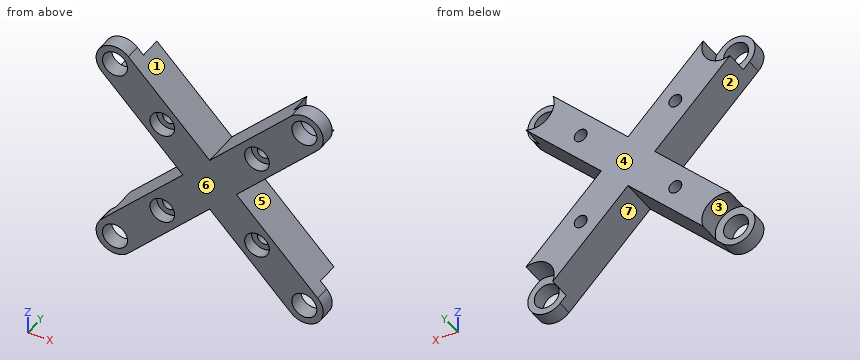
```python
from build123d import *

# Parameters (mm, degrees)
EXTRUDE1_DEPTH                 = 10
CBORE_FOR_M6_SHCS2_D           = 6.6
CBORE_FOR_M6_SHCS2_CBORE_D     = 11
CBORE_FOR_M6_SHCS2_CBORE_DEPTH = 6
LPATTERN1_COUNT                = 2
LPATTERN1_PITCH                = 50
LPATTERN1_COUNT_DIR2           = 2
LPATTERN1_PITCH_DIR2           = 50
CBORE_FOR_M3_SHCS1_D           = 3.4
CBORE_FOR_M3_SHCS1_CBORE_D     = 6.5
CBORE_FOR_M3_SHCS1_CBORE_DEPTH = 3
LPATTERN2_COUNT                = 2
LPATTERN2_PITCH                = 25
LPATTERN2_COUNT_DIR2           = 2
LPATTERN2_PITCH_DIR2           = 25


with BuildPart() as part:
    # Sketch1 → Extrude1 (new body)
    with BuildSketch(Plane(origin=(0, 0, 0), x_dir=(1, 0, 0), z_dir=(0, 1, 0))):
        with BuildLine():
            Line((7.071067812, 0), (28.535533906, 21.464466094))
            ThreePointArc((28.535533906, 21.464466094), (28.535533906, 28.535533906), (21.464466094, 28.535533906))
            Line((21.464466094, 28.535533906), (0, 7.071067812))
            Line((0, 7.071067812), (-21.464466094, 28.535533906))
            ThreePointArc((-21.464466094, 28.535533906), (-28.535533906, 28.535533906), (-28.535533906, 21.464466094))
            Line((-28.535533906, 21.464466094), (-7.071067812, 0))
            Line((-7.071067812, 0), (-28.535533906, -21.464466094))
            ThreePointArc((-28.535533906, -21.464466094), (-28.535533906, -28.535533906), (-21.464466094, -28.535533906))
            Line((-21.464466094, -28.535533906), (0, -7.071067812))
            Line((0, -7.071067812), (21.464466094, -28.535533906))
            ThreePointArc((21.464466094, -28.535533906), (28.535533906, -28.535533906), (28.535533906, -21.464466094))
            Line((28.535533906, -21.464466094), (7.071067812, 0))
        make_face()
    extrude(amount=EXTRUDE1_DEPTH)

    # CBORE for M6 SHCS2 (through all)
    with Locations(Plane(origin=(-25, 10, -25), x_dir=(0, 0, 1), z_dir=(0, 1, 0))):
        with Locations((0, 0)):
            cbore_for_m6_shcs2 = CounterBoreHole(CBORE_FOR_M6_SHCS2_D / 2, CBORE_FOR_M6_SHCS2_CBORE_D / 2, CBORE_FOR_M6_SHCS2_CBORE_DEPTH)

    # LPattern1: CBORE for M6 SHCS2 2 × 2
    with Locations(*[(i * LPATTERN1_PITCH, 0, j * LPATTERN1_PITCH_DIR2) for i in range(LPATTERN1_COUNT) for j in range(LPATTERN1_COUNT_DIR2) if (i, j) != (0, 0)]):
        add(cbore_for_m6_shcs2, mode=Mode.SUBTRACT)

    # CBORE for M3 SHCS1 (through all)
    with Locations(Plane(origin=(-12.5, 0, 12.5), x_dir=(0, 0, -1), z_dir=(0, -1, 0))):
        with Locations((0, 0)):
            cbore_for_m3_shcs1 = CounterBoreHole(CBORE_FOR_M3_SHCS1_D / 2, CBORE_FOR_M3_SHCS1_CBORE_D / 2, CBORE_FOR_M3_SHCS1_CBORE_DEPTH)

    # LPattern2: CBORE for M3 SHCS1 2 × 2
    with Locations(*[(i * LPATTERN2_PITCH, 0, -j * LPATTERN2_PITCH_DIR2) for i in range(LPATTERN2_COUNT) for j in range(LPATTERN2_COUNT_DIR2) if (i, j) != (0, 0)]):
        add(cbore_for_m3_shcs1, mode=Mode.SUBTRACT)


solid = part.part
```
Model file for the job. Use its own axes, mm. Face numbers are marked on the shaded views. A direction names the side the tool comes from. Coordinates: 2 decimals unless noted, no trailing zeros. Order: outer loops, then holes, each group sorted by start corner. A loop starts at its lowest first (then second) coordinate and runs counter-clockwise, first axis right, second up. Notation, with made-up numbers: (63, 44.25) - (114, 44.25) arc R22 cw to (114, 63.25) - close; hole circle Ø8 at (64.5, -40). An arc over 180 degrees is marked (long way). Return JSON: item names as keys, results as strings. Group by question number.
1) Saw through at D-D, the plane z = -17.5. Write the cut outline in (x, y), plus the area to 3 significant figures.
2) Flat gauge pins, fed straight in: P1, Ø3, axis at x = -27, z = -25.5, coming from the +Y side; P2, Ø5.5, axis at x = 12.5, z = 12.5, coming from the -Y side; P3, Ø1.5, axis at x = 14, y = 6, coming from the +Z side. Where does each tip first touch, or does it go through?
3) Mould opens along X. For the marked faces 5, 6 and 7 say: released by +X, released by -X, zero draft, split by the parting line, or undercut.
4) Probe line 1 (X direction, y = 3.05, z = -25); line 2 (X direction, y = 1.1, z = -12.5); line 3 (Z direction, x = -13, y = 0.5). List the from-to ranges inside material, lowest first. Write a range as from..to.
5) Saw through at B-B, the plane x = 12.5. Write the cut outline in (y, z).
6) Saw through at A-A, the plane z = 25. Write the cut outline in (x, y), plus the area to 3 significant figures.
7) Tool access for the marked faces 1, 2, 3 and 4: list every direction of +Z, -Z, +X, -X, +Y, -Y with a clear straight run to the whole face (end or side of a thin tool).
8) Saw through at C-C, the plane y = 5.5. Write the cut outline in (x, z), plus the area to 3 significant figures.
Values found:
{
 "1": {"outline": "(-24.57, 0) - (-10.43, 0) - (-10.43, 10) - (-24.57, 10) - close; (10.43, 0) - (24.57, 0) - (24.57, 10) - (10.43, 10) - close", "area": "283 mm²"},
 "2": {"P1": "stops at y = 4", "P2": "stops at y = 3", "P3": "stops at z = 21.82"},
 "3": {"face 5": "released by +X", "face 6": "zero draft", "face 7": "undercut"},
 "4": {"line 1": "x = -30..-28.3, -21.7..-17.93, 17.93..21.7, 28.3..30", "line 2": "x = -19.57..-15.75, -9.25..-5.43, 5.43..9.25, 15.75..19.57", "line 3": "z = -20.07..-15.71, -9.29..-5.93, 5.93..9.29, 15.71..20.07"},
 "5": {"outline": "(0, -19.57) - (10, -19.57) - (10, -14.2) - (3, -14.2) - (3, -15.75) - (0, -15.75) - close; (0, -9.25) - (3, -9.25) - (3, -10.8) - (10, -10.8) - (10, -5.43) - (0, -5.43) - close; (0, 5.43) - (10, 5.43) - (10, 10.8) - (3, 10.8) - (3, 9.25) - (0, 9.25) - close; (0, 15.75) - (3, 15.75) - (3, 14.2) - (10, 14.2) - (10, 19.57) - (0, 19.57) - close"},
 "6": {"outline": "(-30, 0) - (-28.3, 0) - (-28.3, 4) - (-30, 4) - close; (-21.7, 0) - (-17.93, 0) - (-17.93, 10) - (-19.5, 10) - (-19.5, 4) - (-21.7, 4) - close; (17.93, 0) - (21.7, 0) - (21.7, 4) - (19.5, 4) - (19.5, 10) - (17.93, 10) - close; (28.3, 0) - (30, 0) - (30, 4) - (28.3, 4) - close", "area": "62.6 mm²"},
 "7": {"face 1": "+Z, +Y, -Y", "face 2": "-X, +Y, -Y", "face 3": "+Y", "face 4": "+Z, -Z, +X, -X, +Y"},
 "8": {"outline": "(-26.92, -19.84) arc R5.5 cw to (-19.84, -26.92) - (0, -7.07) - (19.84, -26.92) arc R5.5 cw to (26.92, -19.84) - (7.07, 0) - (26.92, 19.84) arc R5.5 cw to (19.84, 26.92) - (0, 7.07) - (-19.84, 26.92) arc R5.5 cw to (-26.92, 19.84) - (-7.07, 0) - close; hole circle Ø3.4 at (-12.5, -12.5); hole circle Ø3.4 at (-12.5, 12.5); hole circle Ø3.4 at (12.5, -12.5); hole circle Ø3.4 at (12.5, 12.5)", "area": "1,090 mm²"}
}
